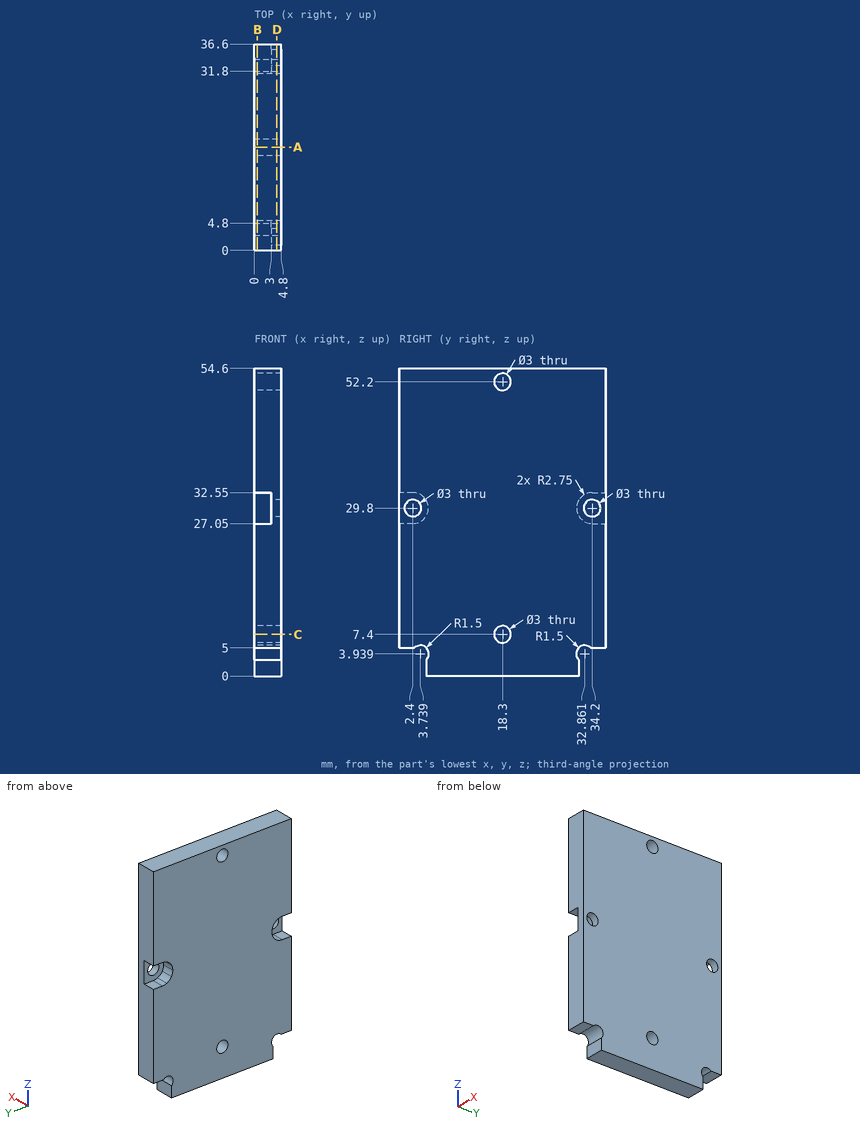
Check sheet for the drawn part. Datum: minimum x, y, z corner. Units: mm. Round coordinates to 2 decimals unless told otherwise and drop trailing zeros. Loops run counter-clockwise (first coordinate to the right, second up) from the corner with the lowest first, then second, coordinate; pieces in that order, holes last. Notation, with made-up numbers: M 83.25,-34 L 103.25,-34 A9 ccw 103.25,-26 Z; hole C 22.5,21 d10. An arc over 180 degrees is marked long. Write each question's results on one line, items separated by ' | '.
1) Scan lines: L1, parallel to Z at x = 1.95, y = 2.5; L2, parallel to Z at x = 2.85, y = 18.3; L3, parallel to Z at x = 4.25, y = 34.2. Record each from-to range of solid material in increasing order. Write a range as from..to.
Checks:
L1: z = 5..27.05, 32.55..54.6 | L2: z = 0..5.9, 8.9..50.7, 53.7..54.6 | L3: z = 5..28.3, 31.3..54.6
2) Section check B-B on x = 0.55. State how many separate pieces and enclosed holes the cut face has, then the cut area to 3 significant figures.
Checks:
separate pieces: 1 | enclosed holes: 2 | area: 1,880 mm2
3) Section check A-A on y = 18.3. Record the boundary of the cut face in (x, z), then the cut area to 3 significant figures.
Checks:
outline: M 0,0 L 4.8,0 L 4.8,5.9 L 0,5.9 Z; M 0,8.9 L 4.8,8.9 L 4.8,50.7 L 0,50.7 Z; M 0,53.7 L 4.8,53.7 L 4.8,54.6 L 0,54.6 Z | area: 233 mm2
4) Section check D-D on x = 4. Record the boundary of the cut face in (y, z).
Checks:
outline: M 0,5 L 2.68,5 A1.5 cw 4.8,2.88 L 4.8,0 L 31.8,0 L 31.8,2.88 A1.5 cw 33.92,5 L 36.6,5 L 36.6,54.6 L 0,54.6 Z; hole C 2.4,29.8 d3; hole C 18.3,7.4 d3; hole C 18.3,52.2 d3; hole C 34.2,29.8 d3
5) Section check C-C on z = 7.4. Record the boundary of the cut face in (x, y), then the cut area to 3 significant figures.
Checks:
outline: M 0,0 L 4.8,0 L 4.8,16.8 L 0,16.8 Z; M 0,19.8 L 4.8,19.8 L 4.8,36.6 L 0,36.6 Z | area: 161 mm2
6) Gauge pin test, flat ends, axial feed: P1, Ø2.5, axis at x = 1, y = 35.5, coming from the -Z side; P2, Ø2.5, axis at y = 1.5, z = 31, coming from the -X side; P3, Ø2.5, axis at x = 3, z = 1, coming from the +Y side; P4, Ø2.5, axis at y = 18.3, z = 7.4, coming from the +X side. Record the tip position at first contact, or that the pin passes through.
Checks:
P1: stops at z = 5 | P2: stops at x = 3 | P3: stops at y = 31.8 | P4: passes through
